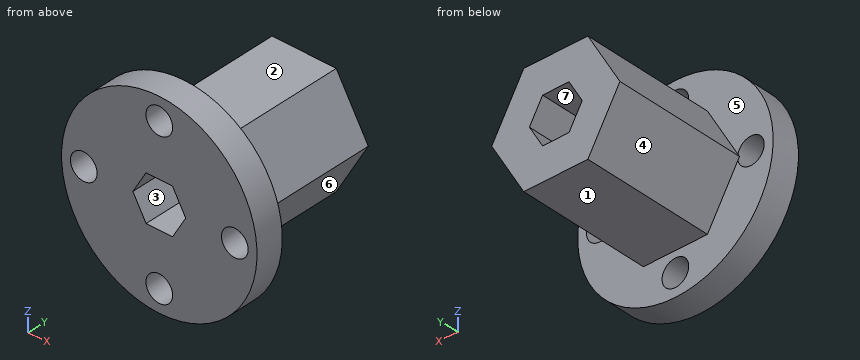
from build123d import *

# Parameters (mm, degrees)
SKETCH1_R           = 11
BOSS_EXTRUDE1_DEPTH = 3.175
BOSS_EXTRUDE2_DEPTH = 15
CUT_EXTRUDE2_DEPTH  = 28
SKETCH6_R           = 1.5
CUT_EXTRUDE3_DEPTH  = 8


with BuildPart() as part:
    # Sketch1 → Boss-Extrude1 (new body)
    with BuildSketch(Plane(origin=(0, 0, 0), x_dir=(1, 0, 0), z_dir=(0, 1, 0))):
        with Locations(Location((0, 0, 0), (0, 0, 270))):
            Circle(SKETCH1_R)
    extrude(amount=BOSS_EXTRUDE1_DEPTH)

    # Sketch2 → Boss-Extrude2 (add)
    with BuildSketch(Plane(origin=(0, 3.175, 0), x_dir=(1, 0, 0), z_dir=(0, 1, 0))):
        Polygon((3.608439182, -6.25), (7.216878365, 0), (3.608439182, 6.25), (-3.608439182, 6.25), (-7.216878365, 0), (-3.608439182, -6.25), align=None)
    extrude(amount=BOSS_EXTRUDE2_DEPTH)

    # Sketch3 → Cut-Extrude2 (cut)
    with BuildSketch(Plane(origin=(0, 18.175, 0), x_dir=(1, 0, 0), z_dir=(0, 1, 0))):
        Polygon((1.486676943, -2.575), (2.973353886, 0), (1.486676943, 2.575), (-1.486676943, 2.575), (-2.973353886, 0), (-1.486676943, -2.575), align=None)
    extrude(amount=-CUT_EXTRUDE2_DEPTH, mode=Mode.SUBTRACT)

    # Sketch6 → Cut-Extrude3 (cut)
    with BuildSketch(Plane(origin=(0, 3.175, 0), x_dir=(1, 0, 0), z_dir=(0, 1, 0))):
        with Locations(Location((0, 8.5, 0), (0, 0, 270))):
            Circle(SKETCH6_R)
        with Locations(Location((8.5, 0, 0), (0, 0, 270))):
            Circle(SKETCH6_R)
        with Locations(Location((0, -8.5, 0), (0, 0, 270))):
            Circle(SKETCH6_R)
        with Locations(Location((-8.5, 0, 0), (0, 0, 270))):
            Circle(SKETCH6_R)
    extrude(amount=-CUT_EXTRUDE3_DEPTH, mode=Mode.SUBTRACT)


solid = part.part
The model under review builds one solid part; all positions refer to its coordinate system, in mm. Face numbers are marked on the shaded views. A direction names the side the tool comes from. Coordinates: 2 decimals unless noted, no trailing zeros. Write each loop counter-clockwise with the first axis right and the second up, starting at its lowest first coordinate (ties: lowest second). Pieces come first, ordered by that corner, then holes. Notation, with made-up numbers: (62.5, -20.75) - (82.5, -20.75) arc R15 ccw to (82.5, -13.75) - close; hole circle Ø1 at (84, 19.25). An arc over 180 degrees is marked (long way). Answer as a JSON object with one key per item and string values. Group by question number.
1. Clearance check with flat-ended pins moving along their axes: pin 1 Ø8 at (x, y) = (8, 8.5) entering from +Z; pin 2 Ø2 at (y, z) = (3.5, -3.5) entering from +X; pin 3 Ø4 at (x, y) = (6.5, 2.5) entering from -Z; pin 4 Ø1.8 at (x, z) = (0, 8.5) entering from +Y. State where each tip first meets the part, or that it passes through.
2. Mouldability with a two-part tool opening along X and no side actions: class the marked faces 5, 6 and 7 as pulls with the +X half, pulls with the -X half, needs draft (parallel to the pull), parting line crosses it, or undercut.
3. Add section C-C (x = 0). Give the boundary of the cut face in (y, z) (3 decimals).
4. Add section B-B (z = 8.5). Give the boundary of the cut face in (x, y) (3 decimals).
5. Add section D-D (x = 8.5). Give the boundary of the cut face in (y, z) (3 decimals).
6. To check wall thickness, follow probe 1 along Z at (x, y) = (0, 17) (3 decimals); probe 2 along Z at (x, y) = (-5.5, 12.25); probe 3 along Z at (x, y) = (-8.5, 2.4). State the ranges of each line that lie inside material, in increasing order.
7. Add section A-A (y = 15). Give the boundary of the cut face in (x, z) (3 decimals), plus the area to 3 significant figures.
8. Machinability: for the marked faces 1, 2, 3 and 4, which of the approach directions +Z, -Z, +X, -X, +Y, -Y give a long, thin tool a straight path to every point of the face, cutting with its end or side? Answer none if there is none.
Findings:
{
 "1": {"pin 1": "z = 5.57", "pin 2": "x = 10.7", "pin 3": "z = -10.04", "pin 4": "through"},
 "2": {"face 5": "needs draft", "face 6": "pulls with the +X half", "face 7": "undercut"},
 "3": {"outline": "(0, -11) - (3.175, -11) - (3.175, -10) - (0, -10) - close; (0, -7) - (3.175, -7) - (3.175, -6.25) - (18.175, -6.25) - (18.175, -2.575) - (0, -2.575) - close; (0, 2.575) - (18.175, 2.575) - (18.175, 6.25) - (3.175, 6.25) - (3.175, 7) - (0, 7) - close; (0, 10) - (3.175, 10) - (3.175, 11) - (0, 11) - close"},
 "4": {"outline": "(-6.982, 0) - (-1.5, 0) - (-1.5, 3.175) - (-6.982, 3.175) - close; (1.5, 0) - (6.982, 0) - (6.982, 3.175) - (1.5, 3.175) - close"},
 "5": {"outline": "(0, -6.982) - (3.175, -6.982) - (3.175, -1.5) - (0, -1.5) - close; (0, 1.5) - (3.175, 1.5) - (3.175, 6.982) - (0, 6.982) - close"},
 "6": {"probe 1": "-6.25 to -2.575, 2.575 to 6.25", "probe 2": "-2.97 to 2.97", "probe 3": "-6.98 to -1.5, 1.5 to 6.98"},
 "7": {"outline": "(-7.217, 0) - (-3.608, -6.25) - (3.608, -6.25) - (7.217, 0) - (3.608, 6.25) - (-3.608, 6.25) - close; hole (-2.973, 0) - (-1.487, -2.575) - (1.487, -2.575) - (2.973, 0) - (1.487, 2.575) - (-1.487, 2.575) - close", "area": "112 mm²"},
 "8": {"face 1": "-Z, +X, -X, +Y", "face 2": "+Z, +X, -X, +Y", "face 3": "+Y, -Y", "face 4": "-Z, -X, +Y"}
}
